For this review, take the finished solid that the model builds, in its own axes (mm). A direction names the side the tool comes from. Round coordinates to 2 decimals unless told otherwise and drop trailing zeros. Write each loop counter-clockwise with the first axis right and the second up, starting at its lowest first coordinate (ties: lowest second). Pieces come first, ordered by that corner, then holes. Notation, with made-up numbers: (62, 65.25) -> (114, 65.25) arc R22 cw to (114, 76.25) -> close; hole circle Ø11 at (6, -38.5). An arc over 180 degrees is marked (long way). Write each question's results on one line, items separated by ' | '. Start each with the question number.
Item 1: Add section B-B (y = -4.5). State the section outline as (x, z) points.
Item 2: The part is to be moulded in two halves that separate along X. For faces 1 (the flat face through (-2.8, -4, -23)), 2 (the cylindrical face through (36.226, 0.986, -22.227)), 3 (the flat face through (152, -3, -36.595)), say which applies: +X half, -X half, draft (parallel to the pull), parting line (faces both ways), or undercut.
Item 3: Clearance check with flat-ended pins moving along their axes: pin 1 (4.5 mm diameter, centred on x = 127.5, z = -5.5, fed in from -Y); pin 2 (5 mm diameter, centred on x = 38, z = -23.15, fed in from +Y); pin 3 (3 mm diameter, centred on x = -1, y = -2, fed in from +Z) (3 decimals); pin 4 (1.4 mm diameter, centred on x = -1.5, y = -1.5, fed in from -Z) (3 decimals). State where each tip first meets the part, or that it passes through.
Item 4: Tool access review of faces 4 (the cylindrical face through (-1.38, -4.049, -33.526)), 5 (the flat face through (151, -4, -23)): name each direction out of +Z, -Z, +X, -X, +Y, -Y from which nothing blocks a thin tool from reaching the whole face with its end or side.
Item 5: To check wall thickness, follow line 1 along X through (y, z) = (-3.25, -15.5); line 2 along Y through (x, z) = (125.5, -17); line 3 along X through (y, z) = (0.5, -31). State the ranges of each line that lie inside material, in increasing order.
Item 6: Add section A-A (x = 38). State the section outline as (y, z) points, plus the area to 3 significant figures.
Item 7: Add section D-D (x = 121). State the section outline as (y, z) points.
Item 8: Add section C-C (z = -16). State the section outline as (x, y) points, plus the area to 3 significant figures.
from build123d import *

# Parameters (mm, degrees)
SKETCH1_R           = 2
BOSS_EXTRUDE1_DEPTH = 2
SKETCH2_W           = 2.8
SKETCH2_H           = 27
BOSS_EXTRUDE2_DEPTH = 10
SKETCH3_R           = 1.5
CUT_EXTRUDE1_DEPTH  = 114.824325613
FILLET1_R           = 1.5
FILLET2_R           = 2
SKETCH4_W           = 118.780737261
SKETCH4_H           = 53.902552227
CUT_EXTRUDE2_DEPTH  = 171
SKETCH5_W           = 33.594975397
SKETCH5_H           = 2
BOSS_EXTRUDE3_DEPTH = 25


with BuildPart() as part:
    # Sketch1 → Boss-Extrude1 (new body)
    with BuildSketch(Plane(origin=(0, 0, 0), x_dir=(1, 0, 0), z_dir=(0, 1, 0))):
        Polygon((0, 6), (2, 0), (33, 0), (35, 5.5), (66, 5.5), (68, 0), (99, 0), (101, 6), (101, 39.094975397), (0, 39.094975397), align=None)
        with Locations(Location((9.5, 5.5, 0), (0, 0, 270))):
            Circle(SKETCH1_R, mode=Mode.SUBTRACT)
        with Locations(Location((23.5, 5.5, 0), (0, 0, 270))):
            Circle(SKETCH1_R, mode=Mode.SUBTRACT)
        with Locations(Location((77.5, 5.5, 0), (0, 0, 90))):
            Circle(SKETCH1_R, mode=Mode.SUBTRACT)
        with Locations(Location((91.5, 5.5, 0), (0, 0, 90))):
            Circle(SKETCH1_R, mode=Mode.SUBTRACT)
        with Locations(Location((30, 23.149785568, 0), (0, 0, 270))):
            Circle(SKETCH1_R, mode=Mode.SUBTRACT)
        with Locations(Location((38, 23.149785568, 0), (0, 0, 270))):
            Circle(SKETCH1_R, mode=Mode.SUBTRACT)
        with Locations(Location((63, 23.149785568, 0), (0, 0, 90))):
            Circle(SKETCH1_R, mode=Mode.SUBTRACT)
        with Locations(Location((71, 23.149785568, 0), (0, 0, 90))):
            Circle(SKETCH1_R, mode=Mode.SUBTRACT)
        Polygon((11, 22.094975397), (14, 19.094975397), (22, 19.094975397), (22, 27.094975397), (11, 27.094975397), align=None, mode=Mode.SUBTRACT)
        Polygon((90, 27.094975397), (90, 22.094975397), (87, 19.094975397), (79, 19.094975397), (79, 27.094975397), align=None, mode=Mode.SUBTRACT)
    extrude(amount=BOSS_EXTRUDE1_DEPTH)

    # Sketch2 → Boss-Extrude2 (add)
    with BuildSketch(Plane(origin=(0, 2, 0), x_dir=(1, 0, 0), z_dir=(0, 1, 0))):
        with Locations((-1.4, 23.094975397)):
            Rectangle(SKETCH2_W, SKETCH2_H)
        with Locations((102.4, 23.094975397)):
            Rectangle(SKETCH2_W, SKETCH2_H)
    extrude(amount=-BOSS_EXTRUDE2_DEPTH)

    # Sketch3 → Cut-Extrude1 (cut, through all)
    with BuildSketch(Plane(origin=(103.8, 0, 0), x_dir=(0, 0, -1), z_dir=(1, 0, 0))):
        with Locations((13.094975397, -4.5)):
            Circle(SKETCH3_R)
        with Locations((32.094975397, -4.5)):
            Circle(SKETCH3_R)
    extrude(amount=-CUT_EXTRUDE1_DEPTH, mode=Mode.SUBTRACT)

    # Fillet1
    fillet1_edges = [part.edges().sort_by_distance(p)[0] for p in [
        (-1.4, -8, -9.594975397),
        (-1.4, -8, -36.594975397),
        (0, 1, -9.594975397),
        (0, 1, -6),
        (2, 1, 0),
        (0, 1, -36.594975397),
        (102.4, -8, -36.594975397),
        (101, 1, -36.594975397),
        (102.4, -8, -9.594975397),
        (101, 1, -9.594975397),
        (101, 1, -6),
        (99, 1, 0),
        (66, 1, -5.5),
        (68, 1, 0),
        (90, 1, -27.094975397),
        (79, 1, -27.094975397),
        (90, 1, -22.094975397),
        (87, 1, -19.094975397),
        (79, 1, -19.094975397),
        (35, 1, -5.5),
        (33, 1, 0),
        (11, 1, -27.094975397),
        (11, 1, -22.094975397),
        (14, 1, -19.094975397),
        (22, 1, -19.094975397),
        (22, 1, -27.094975397),
    ]]
    fillet(fillet1_edges, radius=FILLET1_R)

    # Fillet2
    fillet2_edges = [part.edges().sort_by_distance(p)[0] for p in [
        (-2.8, 2, -23.094975397),
        (103.8, 2, -23.094975397),
    ]]
    fillet(fillet2_edges, radius=FILLET2_R)

    # Sketch4 → Cut-Extrude2 (cut)
    with BuildSketch(Plane(origin=(50.5, 0, 0), x_dir=(0, 0, -1), z_dir=(1, 0, 0))):
        with Locations((-7.200535956, 8.280511496)):
            Rectangle(SKETCH4_W, SKETCH4_H)
    extrude(amount=CUT_EXTRUDE2_DEPTH, mode=Mode.SUBTRACT)

    # Sketch5 → Boss-Extrude3 (add)
    with BuildSketch(Plane(origin=(50.5, 0, 0), x_dir=(0, 0, -1), z_dir=(1, 0, 0))):
        with Locations((22.297487698, 1)):
            Rectangle(SKETCH5_W, SKETCH5_H)
    extrude(amount=BOSS_EXTRUDE3_DEPTH)

    # Mirror1: part across plane


with BuildPart() as part_1:
    add(part.part)
    add(part.part.mirror(Plane(origin=(75.5, 0, 0), x_dir=(0, 0, 1), z_dir=(1, 0, 0))))


solid = part_1.part
Responses:
1) outline: (-2.8, -36.59) -> (0, -36.59) -> (0, -33.59) -> (-2.8, -33.59) -> close; (-2.8, -30.59) -> (0, -30.59) -> (0, -14.59) -> (-2.8, -14.59) -> close; (-2.8, -11.59) -> (0, -11.59) -> (0, -9.59) -> (-2.8, -9.59) -> close; (151, -36.59) -> (153.8, -36.59) -> (153.8, -33.59) -> (151, -33.59) -> close; (151, -30.59) -> (153.8, -30.59) -> (153.8, -14.59) -> (151, -14.59) -> close; (151, -11.59) -> (153.8, -11.59) -> (153.8, -9.59) -> (151, -9.59) -> close
2) face 1: -X half | face 2: undercut | face 3: draft
3) pin 1: stops at y = 0 | pin 2: stops at y = 2 | pin 3: stops at z = -9.595 | pin 4: stops at z = -36.595
4) face 4: +X, -X | face 5: +Z, -Z, -Y
5) line 1: x = -2.8 to 0, 151 to 153.8 | line 2: y = 0 to 2 | line 3: x = -2.74 to 153.74
6) outline: (0, -39.09) -> (2, -39.09) -> (2, -25.15) -> (0, -25.15) -> close; (0, -21.15) -> (2, -21.15) -> (2, -5.5) -> (0, -5.5) -> close | area: 59.2 mm^2
7) outline: (0, -39.09) -> (2, -39.09) -> (2, -25.15) -> (0, -25.15) -> close; (0, -21.15) -> (2, -21.15) -> (2, 0) -> (0, 0) -> close
8) outline: (-2.8, -8) -> (0, -8) -> (0, 0) -> (151, 0) -> (151, -8) -> (153.8, -8) -> (153.8, 0) arc R2 ccw to (151.8, 2) -> (-0.8, 2) arc R2 ccw to (-2.8, 0) -> close | area: 356 mm^2
